from build123d import *

# Parameters (mm, degrees)
SKETCH_1_R          = 1.6
EXTRUDE_1_DEPTH     = 3
FILLET_1_R          = 0.5
FILLET_2_R          = 1
SKETCH_2_R          = 2.5
SKETCH_2_R_2        = 2
CUT_EXTRUDE_1_DEPTH = 76.782265655


with BuildPart() as part:
    # ｽｹｯﾁ1 → ﾎﾞｽ - 押し出し1 (new body)
    with BuildSketch(Plane.XY):
        with BuildLine():
            Line((-47.808090415, -32.754468565), (27.492971995, -32.754468565))
            ThreePointArc((27.492971995, -32.754468565), (30.96632686, -35.823416389), (28.348513235, -39.64829372))
            Line((28.348513235, -39.64829372), (-34.86772632, -55.584323858))
            ThreePointArc((-34.86772632, -55.584323858), (-36.882286825, -55.493024152), (-38.512072834, -54.305342702))
            Line((-38.512072834, -54.305342702), (-50.596895689, -38.369312564))
            ThreePointArc((-50.596895689, -38.369312564), (-50.942731861, -34.697541141), (-47.808090415, -32.754468565))
        make_face()
        with Locations((-47.808090415, -36.254468565)):
            Circle(SKETCH_1_R, mode=Mode.SUBTRACT)
        with Locations((27.492971995, -36.254468565)):
            Circle(SKETCH_1_R, mode=Mode.SUBTRACT)
        with Locations((-35.72326756, -52.190498703)):
            Circle(SKETCH_1_R, mode=Mode.SUBTRACT)
        Polygon((-40.761361774, -39.754468565), (-0.709511909, -39.754468565), (-34.333570517, -48.230676816), align=None, mode=Mode.SUBTRACT)
    extrude(amount=EXTRUDE_1_DEPTH)

    # ﾌｨﾚｯﾄ1
    fillet_1_edges = [part.edges().sort_by_distance(p)[0] for p in [
        (-0.709511909, -39.754468565, 1.5),
    ]]
    fillet(fillet_1_edges, radius=FILLET_1_R)

    # ﾌｨﾚｯﾄ2
    fillet_2_edges = [part.edges().sort_by_distance(p)[0] for p in [
        (-40.761361774, -39.754468565, 1.5),
        (-34.333570517, -48.230676816, 1.5),
    ]]
    fillet(fillet_2_edges, radius=FILLET_2_R)

    # ｽｹｯﾁ2 → ｶｯﾄ - 押し出し1 (cut, through all)
    with BuildSketch(Plane.XY.offset(3)):
        with Locations((7.159021017, -38.858395913)):
            Circle(SKETCH_2_R)
        with Locations((18.069921542, -37.461166604)):
            Circle(SKETCH_2_R_2)
    extrude(amount=-CUT_EXTRUDE_1_DEPTH, mode=Mode.SUBTRACT)


solid = part.part
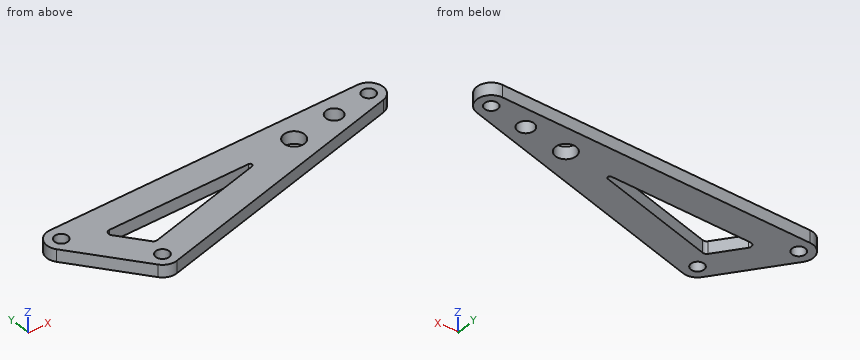
Input: part model. Units: mm. Frame: model coordinates. Round coordinates to 2 decimals unless told otherwise and drop trailing zeros. Loops run counter-clockwise (first coordinate to the right, second up) from the corner with the lowest first, then second, coordinate; pieces in that order, holes last. Notation, with made-up numbers: (80, -39) -> (127, -39) arc R9 cw to (127, -32) -> close; hole circle Ø2 at (88.25, 87). An arc over 180 degrees is marked (long way). Answer as a JSON object with one key per item and string values. Group by question number.
1) Section query C-C on y = -53. Output: boundary loops of the cut face in (x, z).
2) Ray query, L1, parallel to X at y = -39.25, z = 1.15; L2, parallel to X at y = -36, z = 1.45; L3, parallel to Y at x = -34.5, z = 1.65. Return the intervals inside material, ascending.
3) Section query B-B on z = 0.95. Output: boundary loops of the cut face in (x, y), plus the area to 3 significant figures.
4) Section query A-A on x = 5.5. Output: boundary loops of the cut face in (y, z).
5) Section query D-D on x = 22. Output: boundary loops of the cut face in (y, z), plus the area to 3 significant figures.
6) Pin query (flat end, axial travel): pin 1 (1.5 mm diameter, centred on x = -20, z = 1, fed in from -Y). Return the tip coordinate at first contact, or that it passes through.
Reply:
{
 "1": {"outline": "(-39.5, 0) -> (-37.1, 0) -> (-37.1, 3) -> (-39.5, 3) -> close; (-34.34, 0) -> (-24.62, 0) -> (-24.62, 3) -> (-34.34, 3) -> close"},
 "2": {"L1": "x = -49.93 to 4.69, 9.63 to 17.18, 18.96 to 29.3", "L2": "x = -51.3 to -49.39, -46.23 to 16.7, 19.44 to 25.91, 29.07 to 30.98", "L3": "y = -55.49 to -53.22, -51.16 to -47.93, -39.75 to -32.75"},
 "3": {"outline": "(-50.6, -38.37) -> (-38.51, -54.31) arc R3.5 ccw to (-34.87, -55.58) -> (28.35, -39.65) arc R3.5 ccw to (27.49, -32.75) -> (-47.81, -32.75) arc R3.5 ccw to start; hole circle Ø3.2 at (-47.81, -36.25); hole (-39.54, -41.36) -> (-34.73, -47.7) arc R1 ccw to (-33.69, -48.07) -> (-4.62, -40.74) arc R0.5 ccw to (-4.74, -39.75) -> (-38.75, -39.75) arc R1 ccw to start; hole circle Ø3.2 at (-35.72, -52.19); hole circle Ø5 at (7.16, -38.86); hole circle Ø4 at (18.07, -37.46); hole circle Ø3.2 at (27.49, -36.25)", "area": "977 mm2"},
 "4": {"outline": "(-45.41, 0) -> (-40.73, 0) -> (-40.73, 3) -> (-45.41, 3) -> close; (-36.99, 0) -> (-32.75, 0) -> (-32.75, 3) -> (-36.99, 3) -> close"},
 "5": {"outline": "(-41.25, 0) -> (-32.75, 0) -> (-32.75, 3) -> (-41.25, 3) -> close", "area": "25.5 mm2"},
 "6": {"pin 1": "stops at y = -52.03"}
}
